The model under review builds one solid part; all positions refer to its coordinate system, in mm. Face numbers are marked on the shaded views. Coordinates: 2 decimals unless noted, no trailing zeros. Write each loop counter-clockwise with the first axis right and the second up, starting at its lowest first coordinate (ties: lowest second). Pieces come first, ordered by that corner, then holes.
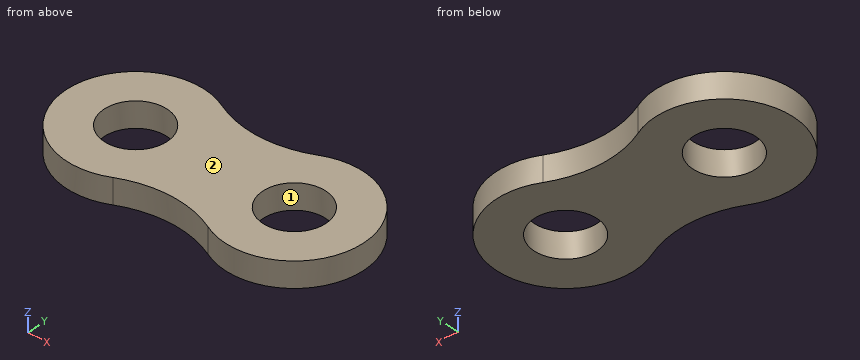
Autodesk Inventor part; units mm, degrees
ref_plane "YZ Plane" through (0, 0, 0) normal (1, 0, 0) x (0, 1, 0)
ref_plane "XZ Plane" through (0, 0, 0) normal (0, 1, 0) x (-1, 0, 0)
ref_plane "XY Plane" through (0, 0, 0) normal (0, 0, 1) x (1, 0, 0)
sketch "Sketch1" plane through (0, 0, 0) normal (0, 0, 1) x (1, 0, 0)
  line L0 (-6.3, 0) -> (6.3, 0) construction
  circle A0 centre (-6.3, 0) radius 2.5
  circle A1 centre (6.3, 0) radius 2.5
  arc A2 (-3.7701, 4.8836) -> (-3.7701, -4.8836) centre (-6.3, 0) ccw
  arc A3 (3.7701, -4.8836) -> (3.7701, 4.8836) centre (6.3, 0) ccw
  line L1 (0, 0) -> (0, 4) construction
  line L2 (0, 0) -> (0, -4) construction
  arc A4 (-3.7701, 4.8836) -> (3.7701, 4.8836) centre (0, 12.4848) ccw
  arc A5 (3.7701, -4.8836) -> (-3.7701, -4.8836) centre (0, -12.4848) ccw
  dimension "d0" = 12.6
  dimension "d1" = 5
  dimension "d2" = 5
  dimension "d3" = 11
  dimension "d4" = 11
  dimension "d5" = 4
  dimension "d6" = 4
extrude "Extrusion1" add sketch "Sketch1" along normal blind 2
properties part number "Concha2"
Item 1: Take a section at C-C, the plane z = 0.65. Write out the cut boundary in (x, y), plus the area to 3 significant figures.
Solved:
outline: (-3.77, -4.88) arc R8.48 cw to (3.77, -4.88) arc R5.5 ccw (long way) to (3.77, 4.88) arc R8.48 cw to (-3.77, 4.88) arc R5.5 ccw (long way) to start; hole circle Ø5 at (-6.3, 0); hole circle Ø5 at (6.3, 0)
area: 174 mm2
Item 2: To check wall thickness, follow line 1 along Y through (x, z) = (6.3, 0.85); line 2 along X through (y, z) = (1, 0.55); line 3 along Y through (x, z) = (-7, 1.85). State the ranges of each line that lie inside material, in increasing order.
Solved:
line 1: y = -5.5 to -2.5, 2.5 to 5.5
line 2: x = -11.71 to -8.59, -4.01 to 4.01, 8.59 to 11.71
line 3: y = -5.46 to -2.4, 2.4 to 5.46
Item 3: Take a section at D-D, the plane x = -6.3. Write out the cut boundary in (y, z), plus the area to 3 significant figures.
Solved:
outline: (-5.5, 0) - (-2.5, 0) - (-2.5, 2) - (-5.5, 2) - close; (2.5, 0) - (5.5, 0) - (5.5, 2) - (2.5, 2) - close
area: 12.0 mm2
Item 4: Take a section at B-B, the plane x = 4.5. Write out the cut boundary in (y, z).
Solved:
outline: (-5.2, 0) - (-1.73, 0) - (-1.73, 2) - (-5.2, 2) - close; (1.73, 0) - (5.2, 0) - (5.2, 2) - (1.73, 2) - close
Item 5: Mouldability with a two-part tool opening along X and no side actions: class the marked faces 1 and 2 as pulls with the +X half, pulls with the -X half, needs draft (parallel to the pull), parting line crosses it, or undercut.
Solved:
face 1: undercut
face 2: needs draft
Item 6: Take a section at A-A, the plane y = 0. Write out the cut boundary in (x, z).
Solved:
outline: (-11.8, 0) - (-8.8, 0) - (-8.8, 2) - (-11.8, 2) - close; (-3.8, 0) - (3.8, 0) - (3.8, 2) - (-3.8, 2) - close; (8.8, 0) - (11.8, 0) - (11.8, 2) - (8.8, 2) - close
